Build history of the part. All positions in model axes, mm. A direction names the side the tool comes from. Give positions to 0.01 mm unless a question says otherwise; leave off trailing zeros. Order: outer loops, then holes, each group sorted by start corner. A loop starts at its lowest first (then second) coordinate and runs counter-clockwise, first axis right, second up. Notation, with made-up numbers: (20.5, 18.5) -> (49.5, 18.5) arc R37 cw to (49.5, 54.5) -> close; hole circle Ø7 at (26, -23.5). An arc over 180 degrees is marked (long way). One line per question, with ' | ' between items. Start each with the question number.
(1) Cut at C-C (y = 235). Give the cut face in (x, z) (3 decimals).
(2) Cut at B-B (x = 173). Give the cut face in (y, z) (3 decimals).
(3) Pin check, flat tips, straight feed: pin 1 Ø15 at (x, z) = (1810, 743) entering from -Y (3 decimals); pin 2 Ø1.9 at (x, y) = (1312.5, -281.5) entering from +Z; pin 3 Ø1.9 at (y, z) = (243.5, -189) entering from +X. Stop position of each tip, or through.
(4) Which spindle directions (+Z, -Z, +X, -X, +Y, -Y) get a long thin tool onto all of the face, cutting with end or side? Do faces 1 (the face through (32, 245, -185.365)), 2 (the face through (1800, -212, 598.005)), 3 (the face through (1800, -153.435, 702)). Say none if no direction does.
(5) Cut at A-A (y = -205). Give the cut face in (x, z) (3 decimals).
(6) Cut at D-D (z = 631). Give the cut face in (x, y) (3 decimals), then the cut area to 3 significant figures.
from build123d import *

# Parameters (mm, degrees)
CROQUIS2_W              = 50.8
CROQUIS2_H              = 570.39
SALIENTE_EXTRUIR1_DEPTH = 6.31
CROQUIS3_W              = 50.8
CROQUIS3_H              = 6.31
SALIENTE_EXTRUIR2_DEPTH = 568.44
CROQUIS4_W              = 50.8
CROQUIS4_H              = 6.31
SALIENTE_EXTRUIR3_DEPTH = 1800
CROQUIS6_W              = 50.8
CROQUIS6_H              = 6.31
CROQUIS9_W              = 50.8
CROQUIS9_H              = 6.31
CROQUIS10_W             = 6.31
CROQUIS10_H             = 50.8
SALIENTE_EXTRUIR4_DEPTH = 65


with BuildPart() as part:
    # Croquis2 → Saliente-Extruir1 (new body)
    with BuildSketch(Plane.XY):
        Rectangle(CROQUIS2_W, CROQUIS2_H)
    extrude(amount=SALIENTE_EXTRUIR1_DEPTH)

    # Croquis3 → Saliente-Extruir2 (add)
    with BuildSketch(Plane.XY.offset(6.31)):
        with Locations((0, -282.04)):
            Rectangle(CROQUIS3_W, CROQUIS3_H)
    extrude(amount=SALIENTE_EXTRUIR2_DEPTH)

    # Croquis4 → Saliente-Extruir3 (add)
    with BuildSketch(Plane(origin=(25.4, 0, 0), x_dir=(0, 0, -1), z_dir=(1, 0, 0))):
        with Locations((-549.35, -282.04)):
            Rectangle(CROQUIS4_W, CROQUIS4_H)
    extrude(amount=SALIENTE_EXTRUIR3_DEPTH)

    # Barrer1: sweep along a curve in space
    with BuildLine() as barrer1_path:
        Line((0, 282.04, 0), (0, 282.04, -188.52))
        Line((0, 282.04, -188.52), (0, 211.24, -188.52))
    # Croquis6 → Barrer1 (sweep)
    with BuildSketch(Plane(origin=(0, 0, 0), x_dir=(-1, 0, 0), z_dir=(0, 0, -1))):
        with Locations((0, 282.04)):
            Rectangle(CROQUIS6_W, CROQUIS6_H)
    sweep(path=barrer1_path.line, transition=Transition.RIGHT)

    # Barrer2: sweep along a curve in space
    with BuildLine() as barrer2_path:
        Line((1800, -282.04, 574.75), (1800, -282.04, 601.16))
        Line((1800, -282.04, 601.16), (1800, -150.28, 601.16))
        Line((1800, -150.28, 601.16), (1800, -150.28, 797.94))
    # Croquis9 → Barrer2 (sweep)
    with BuildSketch(Plane.XY.offset(574.75)):
        with Locations((1800, -282.04)):
            Rectangle(CROQUIS9_W, CROQUIS9_H)
    sweep(path=barrer2_path.line, transition=Transition.RIGHT)

    # Croquis10 → Saliente-Extruir4 (add)
    with BuildSketch(Plane(origin=(25.4, 0, 0), x_dir=(0, 0, -1), z_dir=(1, 0, 0))):
        with Locations((188.52, 236.64)):
            Rectangle(CROQUIS10_W, CROQUIS10_H)
    extrude(amount=SALIENTE_EXTRUIR4_DEPTH)


solid = part.part
Result set:
1) outline: (-25.4, -191.675) -> (90.4, -191.675) -> (90.4, -185.365) -> (-25.4, -185.365) -> close; (-25.4, 0) -> (25.4, 0) -> (25.4, 6.31) -> (-25.4, 6.31) -> close
2) outline: (-285.195, 523.95) -> (-278.885, 523.95) -> (-278.885, 574.75) -> (-285.195, 574.75) -> close
3) pin 1: stops at y = -153.435 | pin 2: stops at z = 574.75 | pin 3: stops at x = 90.4
4) face 1: +X, -X, -Y | face 2: -Z, +X, -X, +Y | face 3: +Z, +X, -X, -Y
5) outline: (-25.4, 0) -> (25.4, 0) -> (25.4, 6.31) -> (-25.4, 6.31) -> close; (1774.6, 598.005) -> (1825.4, 598.005) -> (1825.4, 604.315) -> (1774.6, 604.315) -> close
6) outline: (1774.6, -153.435) -> (1825.4, -153.435) -> (1825.4, -147.125) -> (1774.6, -147.125) -> close | area: 321 mm2
